```python
from build123d import *

# Parameters (mm, degrees)
F1_DEPTH = 63.5
F0_W     = 25.4
F0_H     = 19.05
F2_DEPTH = 25.4
F3_DEPTH = 7.9375


with BuildPart() as f1:
    # F0 (on Front) → F1 (new body, symmetric)
    with BuildSketch(Plane.XZ):
        Polygon((22.225, 9.525), (-41.275, 9.525), (-41.275, -9.525), (41.275, -9.525), (41.275, 9.525), align=None)
    extrude(amount=F1_DEPTH, both=True)

    # F0 (on Front) → F2 (join, symmetric)
    with BuildSketch(Plane.XZ):
        with BuildLine():
            Line((22.225, 24.3588639732), (22.225, 9.525))
            Line((22.225, 9.525), (41.275, 9.525))
            Line((41.275, 9.525), (41.275, 24.3588639732))
            ThreePointArc((41.275, 24.3588639732), (45.9246798487, 35.5841841245), (57.15, 40.2338639732))
            Line((57.15, 40.2338639732), (75.6350584984, 40.2338639732))
            Line((75.6350584984, 40.2338639732), (75.6350584984, 59.2838639732))
            Line((75.6350584984, 59.2838639732), (57.15, 59.2838639732))
            add(Edge.make_bspline(
                [(56.4216107745, 59.2762675727), (56.6651505672, 59.2792783634), (56.9079531463, 59.2818095803), (57.15, 59.2838639732)],
                knots=[109.6042187191, 109.6042187191, 109.6042187191, 109.6042187191, 110.287919415, 110.287919415, 110.287919415, 110.287919415], degree=3))
            ThreePointArc((56.4216107745, 59.2762675727), (32.1981000854, 48.7956869183), (22.225, 24.3588639732))
        make_face()
        with Locations((88.3350584984, 49.7588639732)):
            Rectangle(F0_W, F0_H)
    extrude(amount=F2_DEPTH, both=True)

    # F0 (on Front) → F3 (join, symmetric)
    with BuildSketch(Plane.XZ):
        with BuildLine():
            add(Edge.make_bspline(
                [(-41.275, 9.525), (-40.6081550387, 45.986200262), (17.3796895691, 58.793607011), (56.4216107745, 59.2762675727)],
                knots=[0, 0, 0, 0, 109.6042187191, 109.6042187191, 109.6042187191, 109.6042187191], degree=3))
            Line((-41.275, 9.525), (22.225, 9.525))
            Line((22.225, 9.525), (22.225, 24.3588639732))
            ThreePointArc((22.225, 24.3588639732), (32.1981000854, 48.7956869183), (56.4216107745, 59.2762675727))
        make_face()
    extrude(amount=F3_DEPTH, both=True)

    # F0 (on Front) → F4 (revolve)
    with BuildSketch(Plane.XZ):
        Polygon((101.0350584984, 62.2014122894), (101.0350584984, 59.2838639732), (101.0350584984, 40.2338639732), (101.0350584984, 33.6264122894), (126.4350584984, 33.6264122894), (126.4350584984, 62.2014122894), align=None)
    revolve(axis=Axis((101.0350584984, 0, 47.9139122894), (0, 0, -1)))


solid = f1.part
```
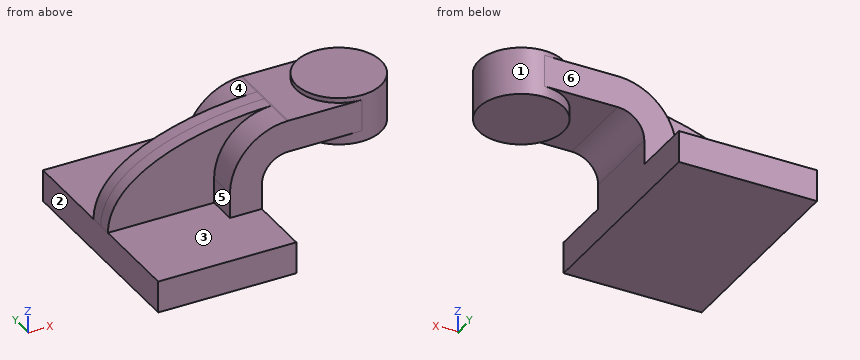
Geometry check sheet. Reference: the model listing, model coordinates, mm. Face numbers are marked on the shaded views. A direction names the side the tool comes from. Coordinates: 2 decimals unless noted, no trailing zeros. Order: outer loops, then holes, each group sorted by start corner. A loop starts at its lowest first (then second) coordinate and runs counter-clockwise, first axis right, second up.
Q1. Tool access check on the marked faces 4, 5 and 6. Record the directions out of +Z, -Z, +X, -X, +Y, -Y that give a thin tool (end or side, any length) a straight path to the whole face; none if there is none.
Reply:
face 4: +Z, -X, +Y
face 5: +Z, -X, -Y
face 6: +Z, +X, -X, +Y
Q2. Sectioned sample at B-B on x = 81.5. Record the cut outline in (y, z).
Reply:
outline: (-25.4, 40.23) - (-16.23, 40.23) - (-16.23, 33.63) - (16.23, 33.63) - (16.23, 40.23) - (25.4, 40.23) - (25.4, 59.28) - (16.23, 59.28) - (16.23, 62.2) - (-16.23, 62.2) - (-16.23, 59.28) - (-25.4, 59.28) - close
Q3. Sectioned sample at A-A on y = 29. Record the cut outline in (x, z) (3 decimals), and give its area (3 significant figures).
Reply:
outline: (-41.275, -9.525) - (41.275, -9.525) - (41.275, 9.525) - (-41.275, 9.525) - close
area: 1,570 mm2
Q4. Depth check by flat-ended pin: pin 1 Ø1.5 at (x, z) = (31.5, 39.5) entering from -Y; pin 2 Ø4.5 at (y, z) = (15, 18) entering from -X (3 decimals); pin 3 Ø25 at (x, z) = (-1, 28) entering from -Y. Enter the tip coordinate at first touch or a pass-through.
Reply:
pin 1: stops at y = -25.4
pin 2: stops at x = 22.225
pin 3: stops at y = -7.94
Q5. Sectioned sample at C-C on z = -1. Record the cut outline in (x, y) (3 decimals), and give its area (3 significant figures).
Reply:
outline: (-41.275, -63.5) - (41.275, -63.5) - (41.275, 63.5) - (-41.275, 63.5) - close
area: 10,500 mm2
Q6. Draft check along X on the marked faces 1, 2 and 3. Enter one of: released by +X, released by -X, zero draft, split by the parting line, or undercut.
Reply:
face 1: undercut
face 2: released by -X
face 3: zero draft
Q7. Thickness scan on probe 1 along Z at (x, y) = (-27, 35) (3 decimals); probe 2 along Y at (x, z) = (41, 51.5); probe 3 along X at (y, z) = (-43, 2) (3 decimals). Record the ranges inside material, lowest first.
Reply:
probe 1: z = -9.525 to 9.525
probe 2: y = -25.4 to 25.4
probe 3: x = -41.275 to 41.275
